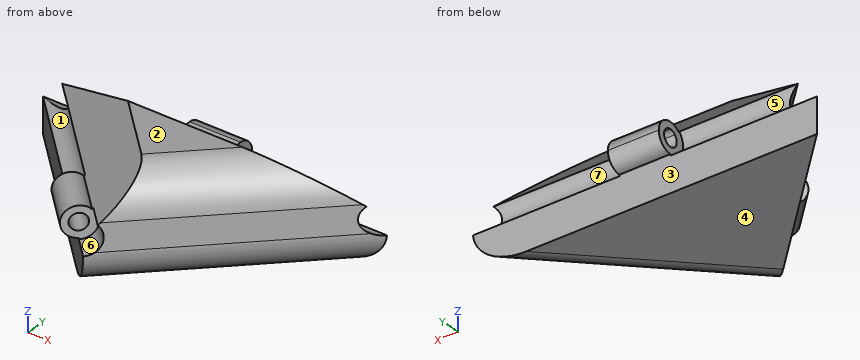
```python
from build123d import *

# Parameters (mm, degrees)
BOSS_EXTRUDE1_DEPTH      = 15
CUT_EXTRUDE1_DEPTH       = 34.582402799
CUT_EXTRUDE1_DEPTH_BACK  = 34.582402799
SKETCH2_R                = 2.4
BOSS_EXTRUDE2_DEPTH      = 3.7
BOSS_EXTRUDE2_DEPTH_BACK = 3.7
SKETCH4_R                = 2.4
SKETCH4_R_2              = 2.2
SKETCH4_R_3              = 1.2
CUT_EXTRUDE2_DEPTH       = 42.134683932
BOSS_EXTRUDE3_START      = -3.8
SKETCH4_3_R              = 1.2
BOSS_EXTRUDE3_DEPTH      = 7.4
FILLET1_R                = 5.5
FILLET2_R                = 5.5


with BuildPart() as part:
    # Sketch1 → Boss-Extrude1 (new body)
    with BuildSketch(Plane(origin=(0, 0, 0), x_dir=(0, 1, 0), z_dir=(0, 0, 1))):
        Polygon((8.333333333, 25), (8.333333333, -25), (-16.666666667, 0), align=None)
    extrude(amount=BOSS_EXTRUDE1_DEPTH)

    # Sketch2 → Cut-Extrude1 (cut, two sides: drawn at the far end of the back side and taken through both)
    with BuildSketch(Plane.YZ.offset(-CUT_EXTRUDE1_DEPTH_BACK)):
        with Locations((8.333333333, 7.5)):
            Circle(SKETCH2_R)
        Polygon((8.333333333, 7.5), (8.333333333, 15), (0.833333333, 15), align=None)
        with BuildLine():
            ThreePointArc((8.333333333, 9.9), (7.414893096, 9.717310878), (6.636277058, 9.197056275))
            Line((6.636277058, 9.197056275), (6.777698415, 9.055634919))
            ThreePointArc((6.777698415, 9.055634919), (7.491429782, 9.532534972), (8.333333333, 9.7))
            Line((8.333333333, 9.7), (8.333333333, 9.9))
        make_face()
        with BuildLine():
            ThreePointArc((8.333333333, 9.7), (7.491429782, 9.532534972), (6.777698415, 9.055634919))
            Line((6.777698415, 9.055634919), (7.484805196, 8.348528137))
            ThreePointArc((7.484805196, 8.348528137), (7.874113214, 8.608655439), (8.333333333, 8.7))
            Line((8.333333333, 8.7), (8.333333333, 9.7))
        make_face()
        with BuildLine():
            Line((7.484805196, 8.348528137), (6.777698415, 9.055634919))
            ThreePointArc((6.777698415, 9.055634919), (6.300798362, 6.658096449), (8.333333333, 5.3))
            ThreePointArc((8.333333333, 5.3), (9.888968252, 5.944365081), (10.533333333, 7.5))
            ThreePointArc((10.533333333, 7.5), (9.888968252, 9.055634919), (8.333333333, 9.7))
            Line((8.333333333, 9.7), (8.333333333, 8.7))
            ThreePointArc((8.333333333, 8.7), (9.181861471, 8.348528137), (9.533333333, 7.5))
            ThreePointArc((9.533333333, 7.5), (7.874113214, 6.391344561), (7.484805196, 8.348528137))
        make_face()
        with BuildLine():
            ThreePointArc((8.333333333, 8.7), (7.874113214, 8.608655439), (7.484805196, 8.348528137))
            Line((7.484805196, 8.348528137), (8.333333333, 7.5))
            Line((8.333333333, 7.5), (8.333333333, 8.7))
        make_face()
        with BuildLine():
            Line((8.333333333, 7.5), (7.484805196, 8.348528137))
            ThreePointArc((7.484805196, 8.348528137), (7.874113214, 6.391344561), (9.533333333, 7.5))
            ThreePointArc((9.533333333, 7.5), (9.181861471, 8.348528137), (8.333333333, 8.7))
            Line((8.333333333, 8.7), (8.333333333, 7.5))
        make_face()
    extrude(amount=CUT_EXTRUDE1_DEPTH + CUT_EXTRUDE1_DEPTH_BACK, mode=Mode.SUBTRACT)

    # Sketch2_5 → Boss-Extrude2 (add, two sides: drawn at the far end of the back side and taken through both)
    with BuildSketch(Plane.YZ.offset(-BOSS_EXTRUDE2_DEPTH_BACK)):
        with BuildLine():
            Line((6.777698415, 9.055634919), (6.636277058, 9.197056275))
            ThreePointArc((6.636277058, 9.197056275), (6.116022455, 6.581559762), (8.333333333, 5.1))
            Line((8.333333333, 5.1), (8.333333333, 5.3))
            ThreePointArc((8.333333333, 5.3), (6.300798362, 6.658096449), (6.777698415, 9.055634919))
        make_face()
        with BuildLine():
            ThreePointArc((8.333333333, 9.7), (7.491429782, 9.532534972), (6.777698415, 9.055634919))
            Line((6.777698415, 9.055634919), (7.484805196, 8.348528137))
            ThreePointArc((7.484805196, 8.348528137), (7.874113214, 8.608655439), (8.333333333, 8.7))
            Line((8.333333333, 8.7), (8.333333333, 9.7))
        make_face()
        with BuildLine():
            Line((7.484805196, 8.348528137), (6.777698415, 9.055634919))
            ThreePointArc((6.777698415, 9.055634919), (6.300798362, 6.658096449), (8.333333333, 5.3))
            ThreePointArc((8.333333333, 5.3), (9.888968252, 5.944365081), (10.533333333, 7.5))
            ThreePointArc((10.533333333, 7.5), (9.888968252, 9.055634919), (8.333333333, 9.7))
            Line((8.333333333, 9.7), (8.333333333, 8.7))
            ThreePointArc((8.333333333, 8.7), (9.181861471, 8.348528137), (9.533333333, 7.5))
            ThreePointArc((9.533333333, 7.5), (7.874113214, 6.391344561), (7.484805196, 8.348528137))
        make_face()
    extrude(amount=BOSS_EXTRUDE2_DEPTH + BOSS_EXTRUDE2_DEPTH_BACK)

    # Sketch4 → Cut-Extrude2 (cut, through all)
    # profile 1 of 3: a face of its own
    with BuildSketch(Plane(origin=(8.333333333, -8.333333333, 0), x_dir=(0.7071067811865486, 0.7071067811865465, 0), z_dir=(0.7071067811865465, -0.7071067811865486, 0))):
        with Locations((-11.78511302, 7.5)):
            Circle(SKETCH4_R)
        with Locations((-11.78511302, 7.5)):
            Circle(SKETCH4_R_2, mode=Mode.SUBTRACT)
    # profile 2 of 3: a face of its own
    with BuildSketch(Plane(origin=(8.333333333, -8.333333333, 0), x_dir=(0.7071067811865486, 0.7071067811865465, 0), z_dir=(0.7071067811865465, -0.7071067811865486, 0))):
        with Locations((-11.78511302, 7.5)):
            Circle(SKETCH4_R_3)
    # profile 3 of 3: a face of its own
    with BuildSketch(Plane(origin=(8.333333333, -8.333333333, 0), x_dir=(0.7071067811865486, 0.7071067811865465, 0), z_dir=(0.7071067811865465, -0.7071067811865486, 0))):
        Polygon((-11.78511302, 7.5), (-4.28511302, 15), (-11.78511302, 15), align=None)
    extrude(amount=-CUT_EXTRUDE2_DEPTH, mode=Mode.SUBTRACT)


with BuildPart() as cut_extrude2_kept_piece:
    # of the separate pieces the step leaves, the one the design keeps (cut_extrude2_pieces_kept)
    add(part.part.solids().sort_by_distance((-25, 8.333333333, 0))[0])

    # Sketch4_3 → Boss-Extrude3 (add)
    with BuildSketch(Plane(origin=(8.333333333, -8.333333333, 0), x_dir=(0.7071067811865486, 0.7071067811865465, 0), z_dir=(0.7071067811865465, -0.7071067811865486, 0)).offset(BOSS_EXTRUDE3_START)):
        with BuildLine():
            Line((-11.78511302, 5.3), (-11.78511302, 5.1))
            ThreePointArc((-11.78511302, 5.1), (-9.567802142, 6.581559762), (-10.088056745, 9.197056275))
            Line((-10.088056745, 9.197056275), (-10.229478101, 9.055634919))
            ThreePointArc((-10.229478101, 9.055634919), (-13.817647991, 8.341903551), (-11.78511302, 5.3))
        make_face()
        with Locations((-11.78511302, 7.5)):
            Circle(SKETCH4_3_R, mode=Mode.SUBTRACT)
    extrude(amount=-BOSS_EXTRUDE3_DEPTH)

    # Fillet1
    fillet1_edges = [cut_extrude2_kept_piece.edges().sort_by_distance(p)[0] for p in [
        (12.5, -4.166666667, 0),
    ]]
    fillet(fillet1_edges, radius=FILLET1_R)

    # Fillet2
    fillet2_edges = [cut_extrude2_kept_piece.edges().sort_by_distance(p)[0] for p in [
        (11.401650429, -5.265016237, 15),
    ]]
    fillet(fillet2_edges, radius=FILLET2_R)


solid = cut_extrude2_kept_piece.part
```
Input: part model. Units: mm. Frame: model coordinates. Face numbers are marked on the shaded views. A direction names the side the tool comes from. Coordinates: 2 decimals unless noted, no trailing zeros. Write each loop counter-clockwise with the first axis right and the second up, starting at its lowest first coordinate (ties: lowest second). Pieces come first, ordered by that corner, then holes. Notation, with made-up numbers: (-36.5, 43.5) - (-4.5, 43.5) arc R21 cw to (-4.5, 70.5) - close; hole circle Ø6 at (-34.75, 65.5). An arc over 180 degrees is marked (long way). Put each result on its own line as item: value. Start each with the question number.
1) Reachability of the marked faces 5, 6 and 7 from +Z, -Z, +X, -X, +Y, -Y: full face, straight path, thin tool, end or side. Return the list, or none.
2) Mould query, pull axis Z, two halves, no side actions, for the marked faces 1, 2, 3 and 4. Classes: pulls with the +Z half, pulls with the -Z half, needs draft (parallel to the pull), parting line crosses it, or undercut.
3) Cut plane A-A (z = 12). Return the cut outline in (x, y), plus the area to 3 significant figures.
4) Contact query for flat-ended pins moving along their axis: pin 1 (3 mm diameter, centred on y = 8.33, z = 7.5, fed in from +X); pin 2 (4 mm diameter, centred on y = -1, z = 4.5, fed in from +X); pin 3 (5 mm diameter, centred on x = -9.5, y = 0.5, fed in from +Z). Output: stop coordinate, or through.
5) Ray query, L1, parallel to Z at x = -2.5, y = 9; L2, parallel to Y at x = 0.5, z = 7.5; L3, parallel to X at y = -12, z = 7. Return the intervals inside material, ascending.
Resolved:
1. face 5: -X, +Y
1. face 6: -Y
1. face 7: +X, +Y
2. face 1: undercut
2. face 2: pulls with the +Z half
2. face 3: needs draft
2. face 4: pulls with the -Z half
3. outline: (-14.14, 3.83) - (2.76, -13.06) - (19.65, 3.83) - close
3. area: 285 mm2
4. pin 1: stops at x = 3.7
4. pin 2: stops at x = 17.58
4. pin 3: stops at z = 14.94
5. L1: z = 5.4 to 6.5, 8.5 to 9.6
5. L2: y = -13.77 to 7.13, 9.53 to 10.53
5. L3: x = -7.7 to -6.21, -3.12 to 4.67
